from build123d import *

# Parameters (mm, degrees)
F0_W     = 304.8
F0_H     = 406.4
F1_DEPTH = 406.4
F3_DEPTH = 609.6
F4_DEPTH = 609.6


with BuildPart() as f1:
    # F0 (on Top) → F1 (new body)
    with BuildSketch(Plane.XY):
        Rectangle(F0_W, F0_H)
    extrude(amount=F1_DEPTH)

    # F2 (on face) → F3 (cut)
    with BuildSketch(Plane(origin=(-152.4, 0, 0), x_dir=(0, -1, 0), z_dir=(-1, 0, 0))):
        Polygon((-167.644607, 0), (-203.2, 406.4), (-203.2, 0), align=None)
    extrude(amount=-F3_DEPTH, mode=Mode.SUBTRACT)

    # F2 (on face) → F4 (cut)
    with BuildSketch(Plane(origin=(-152.4, 0, 0), x_dir=(0, -1, 0), z_dir=(-1, 0, 0))):
        Polygon((203.2, 0), (203.2, 406.4), (167.644607, 0), align=None)
    extrude(amount=-F4_DEPTH, mode=Mode.SUBTRACT)


solid = f1.part
Model file for the job. Use its own axes, mm. Give positions to 0.01 mm unless a question says otherwise; leave off trailing zeros. Loops run counter-clockwise (first coordinate to the right, second up) from the corner with the lowest first, then second, coordinate; pieces in that order, holes last.
1) Wall check: line 1 (Y direction, x = -24, z = 291); line 2 (Y direction, x = -55, z = 169). Give the ranges that are in metal, low to high.
2) Saw through at B-B (z = 124). Write the cut outline in (x, y).
3) Flat gauge pins, fed straight in: pin 1 Ø10 at (x, z) = (100.5, 125.5) entering from -Y; pin 2 Ø3 at (x, z) = (-113, 182.5) entering from -Y; pin 3 Ø2 at (x, z) = (-68.5, 251) entering from -Y. Where does each tip first touch, or does it go through?
4) Saw through at A-A (x = -116). Write the cut outline in (y, z), plus the area to 3 significant figures.
Answer block:
1. line 1: y = -193.1 to 193.1
1. line 2: y = -182.43 to 182.43
2. outline: (-152.4, -178.49) - (152.4, -178.49) - (152.4, 178.49) - (-152.4, 178.49) - close
3. pin 1: stops at y = -179.06
3. pin 2: stops at y = -183.74
3. pin 3: stops at y = -189.69
4. outline: (-203.2, 406.4) - (-167.64, 0) - (167.64, 0) - (203.2, 406.4) - close
4. area: 151,000 mm2
